Here's how the part is built. I have some questions about the finished solid (model axes, mm). Face numbers are marked on the shaded views. A direction names the side the tool comes from. Coordinates: 2 decimals unless noted, no trailing zeros. Loops run counter-clockwise (first coordinate to the right, second up) from the corner with the lowest first, then second, coordinate; pieces in that order, holes last. Notation, with made-up numbers: (60.5, -28.5) - (100.5, -28.5) arc R9 ccw to (100.5, -20.5) - close; hole circle Ø9 at (-40, -9.75). An arc over 180 degrees is marked (long way). Use a Markdown table: item, result.
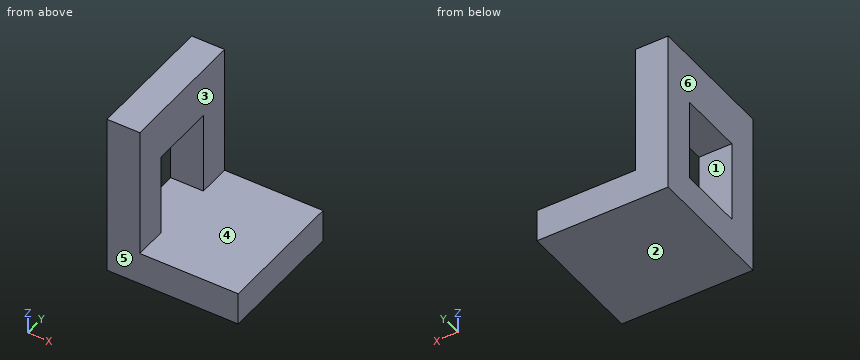
```python
from build123d import *

# Parameters (mm, degrees)
F1_DEPTH = 20
F2_W     = 20
F2_H     = 25
F3_DEPTH = 25.4


with BuildPart() as f1:
    # F0 (on Front) → F1 (new body, symmetric)
    with BuildSketch(Plane.XZ):
        Polygon((0, 0), (0, 10), (-30, 10), (-30, 50), (-40, 50), (-40, 0), align=None)
    extrude(amount=F1_DEPTH, both=True)

    # F2 (on face) → F3 (cut)
    with BuildSketch(Plane.YZ.offset(-30)):
        with Locations((0, 22.5)):
            Rectangle(F2_W, F2_H)
    extrude(amount=-F3_DEPTH, mode=Mode.SUBTRACT)


solid = f1.part
```
Q1. If we mould it in two halves opening along Y, with no side actions, what happens to the marked faces 4, 5 and 6? For each: pulls with the +Y half, pulls with the -Y half, needs draft (parallel to the pull), parting line crosses it, or undercut.
Check values:
| item | result |
|---|---|
| face 4 | undercut |
| face 5 | pulls with the -Y half |
| face 6 | needs draft |
Q2. I want a section at B-B, the plane z = 25. Write out the boundary of the cut face in (x, y).
Check values:
| item | result |
|---|---|
| outline | (-40, -20) - (-30, -20) - (-30, -10) - (-40, -10) - close; (-40, 10) - (-30, 10) - (-30, 20) - (-40, 20) - close |
Q3. I want a section at D-D, the plane y = 16.5. Write out the boundary of the cut face in (x, z).
Check values:
| item | result |
|---|---|
| outline | (-40, 0) - (0, 0) - (0, 10) - (-30, 10) - (-30, 50) - (-40, 50) - close |
Q4. Which directions (+Z, -Z, +X, -X, +Y, -Y) give clear straight access to the entire face, cutting with the end or side of a thin tool? Please do the marked faces 1, 2 and 3.
Check values:
| item | result |
|---|---|
| face 1 | +X, -X |
| face 2 | -Z, +X, -X, +Y, -Y |
| face 3 | +Z, +X, +Y, -Y |
Q5. Please list where these lines run through material, in increasing order: L1, parallel to X at y = -7.5, z = 47.5; L2, parallel to Z at x = -4, y = 17.5. Write a range as from..to.
Check values:
| item | result |
|---|---|
| L1 | -40..-30 |
| L2 | 0..10 |
Q6. I want a section at C-C, the plane x = -24. Write out the boundary of the cut face in (y, z).
Check values:
| item | result |
|---|---|
| outline | (-20, 0) - (20, 0) - (20, 10) - (-20, 10) - close |
Q7. Will these pins go through, and if not, where does the flat tip stop? P1, Ø8, axis at y = 15.5, z = 20, coming from the +X side; P2, Ø8, axis at x = -32, y = 2.5, coming from the -Z side; P3, Ø12, axis at x = -11.5, y = 6.5, coming from the +Z side.
Check values:
| item | result |
|---|---|
| P1 | x = -30 |
| P2 | z = 0 |
| P3 | z = 10 |
Q8. I want a section at A-A, the plane y = -9. Write out the boundary of the cut face in (x, z).
Check values:
| item | result |
|---|---|
| outline | (-40, 0) - (0, 0) - (0, 10) - (-40, 10) - close; (-40, 35) - (-30, 35) - (-30, 50) - (-40, 50) - close |
